Read the model definition and answer for the solid it produces. Units are mm, in the model's axes. Face numbers are marked on the shaded views. A direction names the side the tool comes from. Round coordinates to 2 decimals unless told otherwise and drop trailing zeros. Loops run counter-clockwise (first coordinate to the right, second up) from the corner with the lowest first, then second, coordinate; pieces in that order, holes last. Notation, with made-up numbers: M 82,-5 L 132,-5 A20 ccw 132,4 Z; hole C 63,-28.5 d1. An arc over 180 degrees is marked long. Write each question's results on one line, items separated by ' | '.
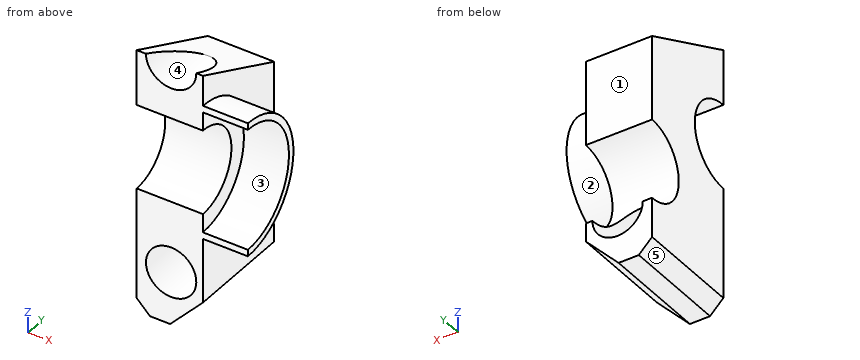
```python
from build123d import *

# Parameters (mm, degrees)
SALIENTE_EXTRUIR1_DEPTH    = 25
CORTAR_EXTRUIR1_DEPTH      = 54
CORTAR_EXTRUIR1_DEPTH_BACK = 94
CROQUIS2_R                 = 9.5
CORTAR_EXTRUIR2_DEPTH      = 94
CORTAR_EXTRUIR2_DEPTH_BACK = 94
CROQUIS3_R                 = 15
CROQUIS3_R_2               = 16
CORTAR_EXTRUIR3_DEPTH      = 94
CORTAR_EXTRUIR3_DEPTH_BACK = 94
CHAFL_N2_SIZE              = 5
SALIENTE_EXTRUIR2_DEPTH    = 17


with BuildPart() as part:
    # Croquis1 → Saliente-Extruir1 (new body)
    with BuildSketch(Plane(origin=(0, 0, 0), x_dir=(0, 0, -1), z_dir=(1, 0, 0))):
        Polygon((-100, 0), (-82, 40), (0, 40), (0, 0), align=None)
    extrude(amount=SALIENTE_EXTRUIR1_DEPTH)

    # Croquis2 → Cortar-Extruir1 (cut, two sides: drawn at the far end of the back side and taken through both)
    with BuildSketch(Plane(origin=(0, 40, 0), x_dir=(1, 0, 0), z_dir=(0, 1, 0)).offset(-CORTAR_EXTRUIR1_DEPTH_BACK)):
        with Locations((13, -100)):
            Circle(CROQUIS2_R)
        with Locations(Location((13, -20, 0), (0, 0, 90))):
            Circle(CROQUIS2_R)
    extrude(amount=CORTAR_EXTRUIR1_DEPTH + CORTAR_EXTRUIR1_DEPTH_BACK, mode=Mode.SUBTRACT)

    # Croquis3 → Cortar-Extruir2 (cut, two sides: drawn at the far end of the back side and taken through both)
    with BuildSketch(Plane(origin=(25, 0, 0), x_dir=(0, 0, -1), z_dir=(1, 0, 0)).offset(-CORTAR_EXTRUIR2_DEPTH_BACK)):
        with Locations((-35, 40)):
            Circle(CROQUIS3_R)
        with Locations((-63, 0)):
            Circle(CROQUIS3_R_2)
    extrude(amount=CORTAR_EXTRUIR2_DEPTH + CORTAR_EXTRUIR2_DEPTH_BACK, mode=Mode.SUBTRACT)

    # Croquis4 → Cortar-Extruir3 (cut, two sides: drawn at the far end of the back side and taken through both)
    with BuildSketch(Plane(origin=(0, 40, 0), x_dir=(1, 0, 0), z_dir=(0, 1, 0)).offset(-CORTAR_EXTRUIR3_DEPTH_BACK)):
        Polygon((12.62, 0), (25, -13.066583333), (25, 0), align=None)
    extrude(amount=CORTAR_EXTRUIR3_DEPTH + CORTAR_EXTRUIR3_DEPTH_BACK, mode=Mode.SUBTRACT)

    # Chafl_n2
    chafl_n2_edges = [part.edges().sort_by_distance(p)[0] for p in [
        (0, 20, 0),
    ]]
    chamfer(chafl_n2_edges, length=CHAFL_N2_SIZE)

    # Croquis5 → Saliente-Extruir2 (add)
    with BuildSketch(Plane(origin=(25, 0, 0), x_dir=(0, 0, -1), z_dir=(1, 0, 0))):
        with BuildLine():
            Line((-88.5, 0), (-86, 0))
            ThreePointArc((-86, 0), (-63, 23), (-40, 0))
            Line((-40, 0), (-37.5, 0))
            ThreePointArc((-37.5, 0), (-63, 25.5), (-88.5, 0))
        make_face()
    extrude(amount=SALIENTE_EXTRUIR2_DEPTH)


solid = part.part
```
1. Which of the six approach directions +Z, -Z, +X, -X, +Y, -Y give full straight-line access (tool end or side, diameter ignored) to the marked faces 1 and 2?
Completed:
face 1: +Z, -Z, +X, -X, +Y | face 2: +X, +Y
2. Find section D-D, the plane y = 35. Give the vertices of the cut face in (x, z), then the cut area to 3 significant figures.
Completed:
outline: M 0,5 L 5,0 L 12.62,0 L 25,13.07 L 25,20.86 L 22.46,20.86 A9.5 cw long 3.54,20.86 L 0,20.86 Z; M 0,49.14 L 25,49.14 L 25,84.25 L 0,84.25 Z | area: 1,150 mm2
3. Find section A-A, the plane z = 63. Give the vertices of the cut face in (x, y).
Completed:
outline: M 0,16 L 25,16 L 25,23 L 42,23 L 42,25.5 L 25,25.5 L 25,40 L 0,40 Z
4. Determine the mould class of the marked faces 3, 4 and 5 for opening direction X: released by +X, released by -X, zero draft, split by the parting line, or undercut.
Completed:
face 3: zero draft | face 4: undercut | face 5: released by -X
5. Find section B-B, the plane y = 13.5. Give the vertices of the cut face in (x, z) (3 decimals), then the cut area to 3 significant figures.
Completed:
outline: M 0,5 L 5,0 L 12.62,0 L 25,13.067 L 25,41.367 L 42,41.367 L 42,44.379 L 25,44.379 L 25,54.412 L 0,54.412 Z; M 0,71.588 L 25,71.588 L 25,81.621 L 42,81.621 L 42,84.633 L 25,84.633 L 25,93.925 L 20.304,93.925 A9.5 cw 5.696,93.925 L 0,93.925 Z; hole C 13,20 d19 | area: 1,610 mm2
6. Find the intervals of material crossed by L1, parallel to X at y = 32, z = 20; L2, parallel to Z at x = 8, y = 14; L3, parallel to X at y = 24, z = 41, in increasing order.
Completed:
L1: x = 0 to 3.5, 22.5 to 25 | L2: z = 0 to 11.92, 28.08 to 55.25, 70.75 to 91.92 | L3: x = 0 to 25
7. Find section C-C, the plane x = 8.5. Give the vertices of the cut face in (y, z).
Completed:
outline: M 0,0 L 40,0 L 40,11.63 L 0,11.63 Z; M 0,28.37 L 26.55,28.37 A15 cw 40,50 L 40,82 L 18.59,91.63 L 0,91.63 L 0,79 A16 cw 0,47 Z
8. Given P1, Ø7, axis at y = 9.5, z = 72, coming from the +X side; P2, Ø12, axis at x = 12.5, y = 22.5, coming from the +Z side; P3, Ø4, axis at x = 26, y = 31, coming from the +Z side, each flat-ended and moving along its own axis, determine where each tip first touches the part or whether it passes through.
Completed:
P1: stops at x = 25 | P2: stops at z = 91.78 | P3: stops at z = 86.83
